Here's how the part is built. I have some questions about the finished solid (model axes, mm). Face numbers are marked on the shaded views. A direction names the side the tool comes from. Give positions to 0.01 mm unless a question says otherwise; leave off trailing zeros. Loops run counter-clockwise (first coordinate to the right, second up) from the corner with the lowest first, then second, coordinate; pieces in that order, holes last.
Q1. For the marked faces 1 and 2, which set-ups out of +Z, -Z, +X, -X, +Y, -Y let a thin tool reach every point of the face, with its end or its side?
Q2. Suppose I cut it at C-C (x = 22.5). List the corners of the cut face in (y, z) for me.
Q3. Suppose I cut it at A-A (y = 0.5). List the corners of the cut face in (x, z) for me.
Q4. Suppose I cut it at B-B (z = -2.25). List the corners of the cut face in (x, y) for me.
Q5. Thinking about a two-plate mould opening in X: for the marked faces 3 and 4, which applies, pulls with the +X half, pulls with the -X half, needs draft (parallel to the pull), parting line crosses it, or undercut?
Q6. I need wall thicknesses on probe 1 along Z at (x, y) = (20.5, 1.7); probe 2 along X at (y, z) = (0.1, -3.5); probe 3 along X at (y, z) = (0.6, -3.75). Which ranges of each line are inside material? Lowest first, please.
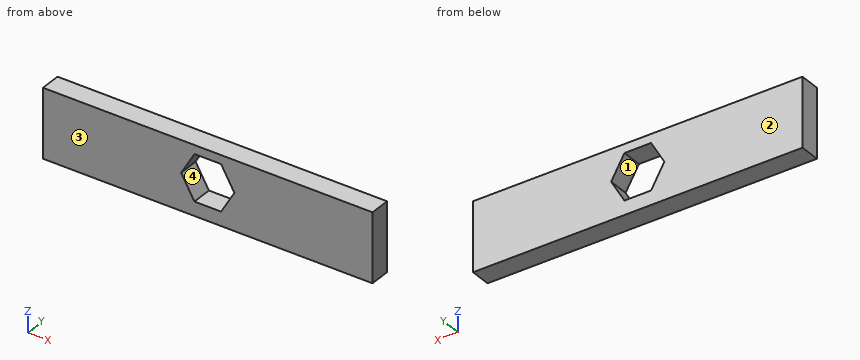
```python
from build123d import *

# Parameters (mm, degrees)
SKIZZE1_W                       = 40
SKIZZE1_H                       = 8.36
AUFSATZ_LINEAR_AUSTRAGEN1_DEPTH = 2.5
SCHNITT_LINEAR_AUSTRAGEN1_DEPTH = 2.5


with BuildPart() as part:
    # Skizze1 → Aufsatz-Linear austragen1 (new body)
    with BuildSketch(Plane(origin=(0, 0, 0), x_dir=(1, 0, 0), z_dir=(0, 1, 0))):
        with Locations((20, 4.18)):
            Rectangle(SKIZZE1_W, SKIZZE1_H)
    extrude(amount=AUFSATZ_LINEAR_AUSTRAGEN1_DEPTH)

    # Skizze3 → Schnitt-Linear austragen1 (cut)
    with BuildSketch(Plane(origin=(0, 2.5, 0), x_dir=(1, 0, 0), z_dir=(0, 1, 0))):
        Polygon((23.233161507, 3.86), (21.616580754, 6.66), (18.383419246, 6.66), (16.766838493, 3.86), (18.383419246, 1.06), (21.616580754, 1.06), align=None)
    extrude(amount=-SCHNITT_LINEAR_AUSTRAGEN1_DEPTH, mode=Mode.SUBTRACT)


solid = part.part
```
Solutions:
1. face 1: +Y, -Y
1. face 2: +Z, -Z, +X, -X, +Y
2. outline: (0, -8.36) - (2.5, -8.36) - (2.5, -5.13) - (0, -5.13) - close; (0, -2.59) - (2.5, -2.59) - (2.5, 0) - (0, 0) - close
3. outline: (0, -8.36) - (40, -8.36) - (40, 0) - (0, 0) - close; hole (16.77, -3.86) - (18.38, -6.66) - (21.62, -6.66) - (23.23, -3.86) - (21.62, -1.06) - (18.38, -1.06) - close
4. outline: (0, 0) - (17.7, 0) - (17.7, 2.5) - (0, 2.5) - close; (22.3, 0) - (40, 0) - (40, 2.5) - (22.3, 2.5) - close
5. face 3: needs draft
5. face 4: undercut
6. probe 1: z = -8.36 to -6.66, -1.06 to 0
6. probe 2: x = 0 to 16.97, 23.03 to 40
6. probe 3: x = 0 to 16.83, 23.17 to 40
